Can you work these out from the model? Positions are in its coordinate system, mm. A direction names the side the tool comes from. Give positions to 0.01 mm unless a question says otherwise; leave off trailing zeros. Loops run counter-clockwise (first coordinate to the right, second up) from the corner with the lowest first, then second, coordinate; pieces in that order, holes last. Notation, with made-up numbers: (49, 4.5) - (92, 4.5) arc R29 cw to (92, 35.5) - close; hole circle Ø1 at (15.25, 74.5). An arc over 180 degrees is marked (long way). Answer as a JSON object with one key per item and string values.
```python
from build123d import *

# Parameters (mm, degrees)
BOSS_EXTRUDE1_DEPTH = 18
SKETCH2_R           = 2.75
CUT_EXTRUDE1_DEPTH  = 18
SKETCH3_R           = 2.75
CUT_EXTRUDE2_DEPTH  = 18


with BuildPart() as part:
    # Sketch1 → Boss-Extrude1 (new body)
    with BuildSketch(Plane.XY):
        Polygon((0, 0), (0, -20.15), (2, -20.15), (2, -2), (20.15, -2), (20.15, 0), align=None)
    extrude(amount=-BOSS_EXTRUDE1_DEPTH)

    # Sketch2 → Cut-Extrude1 (cut)
    with BuildSketch(Plane.XZ.offset(2)):
        with Locations((10.075, -9)):
            Circle(SKETCH2_R)
    extrude(amount=-CUT_EXTRUDE1_DEPTH, mode=Mode.SUBTRACT)

    # Sketch3 → Cut-Extrude2 (cut)
    with BuildSketch(Plane(origin=(2, 0, 0), x_dir=(0, 0, -1), z_dir=(1, 0, 0))):
        with Locations((9, -10.075)):
            Circle(SKETCH3_R)
    extrude(amount=-CUT_EXTRUDE2_DEPTH, mode=Mode.SUBTRACT)


solid = part.part
```
1) I'm going to push flat-ended pins straight in: P1, Ø10, axis at x = 3, y = -14.5, coming from the +Z side; P2, Ø8, axis at y = -16, z = -5.5, coming from the +X side; P3, Ø3.5, axis at x = 10.075, z = -9, coming from the +Y side; P4, Ø5, axis at x = 9, z = -11.5, coming from the -Y side. Where does each tip first touch, or does it pass through?
Check sheet entries:
{"P1": "z = 0", "P2": "x = 2", "P3": "through", "P4": "y = -2"}
2) Which directions (+Z, -Z, +X, -X, +Y, -Y) give clear straight access to the entire face, cutting with the end or side of a thin tool? Please do faces 1 (the flat face through (20.15, -1, -9)), 2 (the flat face through (13, -2, -9)).
Check sheet entries:
{"face 1": "+Z, -Z, +X, +Y, -Y", "face 2": "+Z, -Z, +X, -Y"}
3) Imagine slicing it at B-B on x = 11.5. Write out the boundary of the cut face in (y, z), and give its area (3 significant figures).
Check sheet entries:
{"outline": "(-2, -18) - (0, -18) - (0, -11.35) - (-2, -11.35) - close; (-2, -6.65) - (0, -6.65) - (0, 0) - (-2, 0) - close", "area": "26.6 mm2"}
4) If we mould it in two halves opening along Z, with no side actions, what happens to faces 3 (the cylindrical face through (7.89, -1.01, -10.67)), 4 (the flat face through (1.8, -5.6, 0)), 5 (the cylindrical face through (1.01, -12.76, -8.4)), 6 (the flat face through (12.5, 0, -10.9))? For each: released by +Z, released by -Z, zero draft, split by the parting line, or undercut.
Check sheet entries:
{"face 3": "undercut", "face 4": "released by +Z", "face 5": "undercut", "face 6": "zero draft"}
5) Imagine slicing it at A-A on z = -9. Write out the boundary of the cut face in (x, y) (3 decimals).
Check sheet entries:
{"outline": "(0, -20.15) - (2, -20.15) - (2, -12.825) - (0, -12.825) - close; (0, -7.325) - (2, -7.325) - (2, -2) - (7.325, -2) - (7.325, 0) - (0, 0) - close; (12.825, -2) - (20.15, -2) - (20.15, 0) - (12.825, 0) - close"}
6) Imagine slicing it at C-C on y = -19. Write out the boundary of the cut face in (x, z), and give its area (3 significant figures).
Check sheet entries:
{"outline": "(0, -18) - (2, -18) - (2, 0) - (0, 0) - close", "area": "36.0 mm2"}
7) Imagine slicing it at D-D on z = -12.75. Write out the boundary of the cut face in (x, y).
Check sheet entries:
{"outline": "(0, -20.15) - (2, -20.15) - (2, -2) - (20.15, -2) - (20.15, 0) - (0, 0) - close"}
8) I need wall thicknesses on L1, parallel to Y at x = 1.55, z = -9 (3 decimals); L2, parallel to X at y = -13.5, z = -4; L3, parallel to Y at x = 14.5, z = -2. Which ranges of each line are inside material? Lowest first, please.
Check sheet entries:
{"L1": "-20.15 to -12.825, -7.325 to 0", "L2": "0 to 2", "L3": "-2 to 0"}
